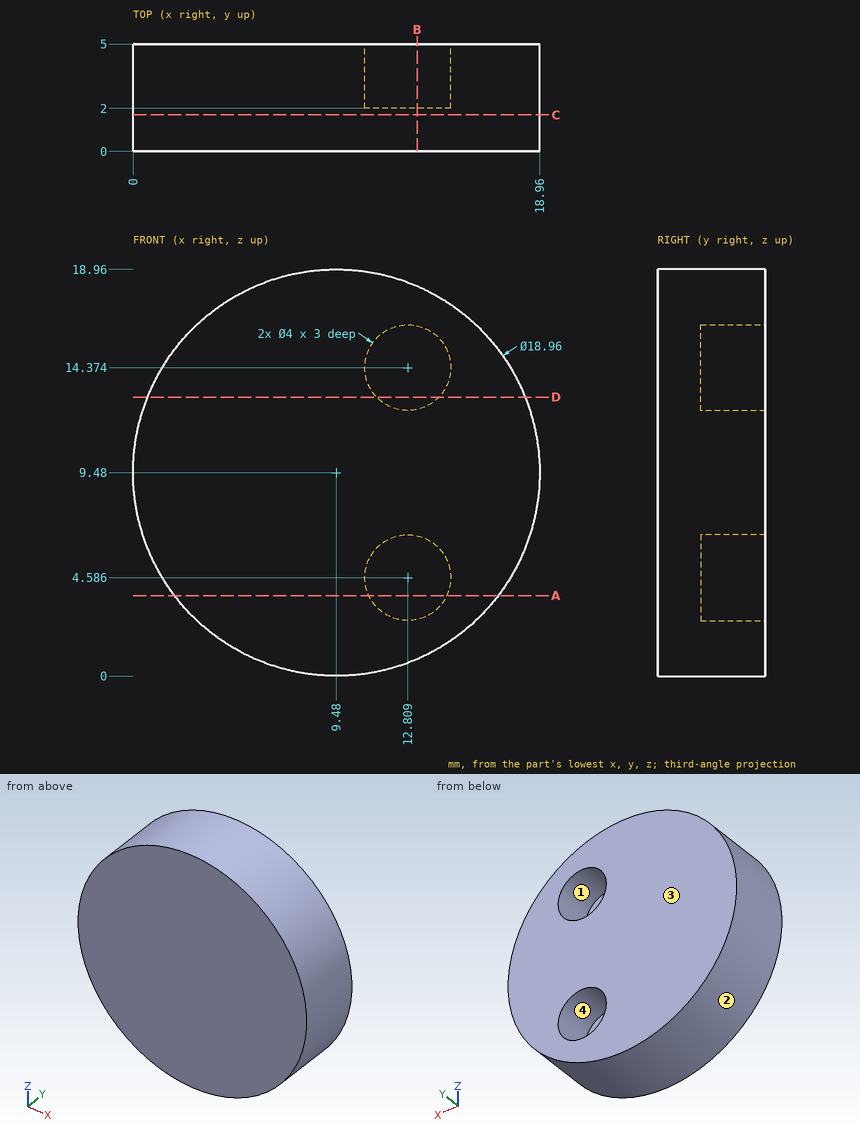
Design review of the part shown in the three views and the two pictorial views. Dimensions are in mm from the part's minimum x, y and z. Coordinates: 2 decimals unless noted, no trailing zeros. Loops run counter-clockwise (first coordinate to the right, second up) from the corner with the lowest first, then second, coordinate; pieces in that order, holes last. Notation, with made-up numbers: (58, 75.5) - (111, 75.5) arc R10 ccw to (111, 80.5) - close; hole circle Ø4 at (52, 14). An arc over 180 degrees is marked (long way). Use a Markdown table: item, result. Add a question column.
Item 1: We need section B-B (x = 13.25). Give the boundary of the cut face in (y, z) (1 decimal).
Item 2: Insertion check: pin 1 Ø1.5 at (x, y) = (11.5, 2) entering from +Z (1 decimal); pin 2 Ø1.2 at (x, z) = (13.5, 4) entering from +Y; pin 3 Ø3 at (x, y) = (4, 1) entering from -Z (1 decimal). Each pin has a flat end and moves straight along its axis. Give the tip position at first contact, or say it passes through.
Item 3: We need section A-A (z = 3.75). Give the boundary of the cut face in (x, y).
Item 4: We need section D-D (z = 13). Give the boundary of the cut face in (x, y).
Item 5: Mouldability with a two-part tool opening along Z and no side actions: class the marked faces 1, 2, 3 and 4 as pulls with the +Z half, pulls with the -Z half, needs draft (parallel to the pull), parting line crosses it, or undercut.
Item 6: We need section C-C (y = 1.7). Give the boundary of the cut face in (x, z).
Item 7: For line 1 (Z direction, x = 11.5, y = 2.55) (1 decimal); line 2 (Z direction, x = 11.25, y = 4.45) (1 decimal); line 3 (X direction, y = 4.3, z = 4.25) (1 decimal), list the stretches that pass through material, from the lowest coordinate up.
Results list:
| question | item | result |
|---|---|---|
| 1 | outline | (0, 0.8) - (5, 0.8) - (5, 2.6) - (2, 2.6) - (2, 6.5) - (5, 6.5) - (5, 12.4) - (2, 12.4) - (2, 16.3) - (5, 16.3) - (5, 18.2) - (0, 18.2) - close |
| 2 | pin 1 | stops at z = 18.9 |
| 2 | pin 2 | stops at y = 2 |
| 2 | pin 3 | stops at z = 0.9 |
| 3 | outline | (1.93, 0) - (17.03, 0) - (17.03, 5) - (14.63, 5) - (14.63, 2) - (10.99, 2) - (10.99, 5) - (1.93, 5) - close |
| 4 | outline | (0.68, 0) - (18.28, 0) - (18.28, 5) - (14.26, 5) - (14.26, 2) - (11.36, 2) - (11.36, 5) - (0.68, 5) - close |
| 5 | face 1 | undercut |
| 5 | face 2 | parting line crosses it |
| 5 | face 3 | needs draft |
| 5 | face 4 | undercut |
| 6 | outline | circle Ø18.96 at (9.48, 9.48) |
| 7 | line 1 | z = 0.2 to 3.1, 6.1 to 12.9, 15.9 to 18.7 |
| 7 | line 2 | z = 0.2 to 3.3, 5.8 to 13.1, 15.6 to 18.8 |
| 7 | line 3 | x = 1.6 to 10.8, 14.8 to 17.4 |
